from build123d import *

# Parameters (mm, degrees)
F1_DEPTH = 14.2875
F3_DEPTH = 28.576
F5_DEPTH = 38.1
F6_R     = 5.08
F7_SIZE  = 2.38125


with BuildPart() as f1:
    # F0 (on Front) → F1 (new body, symmetric)
    with BuildSketch(Plane.XZ):
        with BuildLine():
            Line((76.2, 14.2875), (41.275, 14.2875))
            Line((41.275, 14.2875), (4.333811, 1.500165))
            ThreePointArc((4.333811, 1.500165), (3.265599, 0), (4.333811, -1.500165))
            Line((4.333811, -1.500165), (41.275, -14.2875))
            Line((41.275, -14.2875), (76.2, -14.2875))
            Line((76.2, -14.2875), (114.3, -14.2875))
            Line((114.3, -14.2875), (114.3, 14.2875))
            Line((114.3, 14.2875), (76.2, 14.2875))
        make_face()
    extrude(amount=F1_DEPTH, both=True)

    # F2 (on face) → F3 (cut, through all)
    with BuildSketch(Plane.XY.offset(14.2875)):
        with BuildLine():
            Line((66.675, 6.35), (53.975, 6.35))
            ThreePointArc((53.975, 6.35), (47.625, 0), (53.975, -6.35))
            Line((53.975, -6.35), (66.675, -6.35))
            ThreePointArc((66.675, -6.35), (73.025, 0), (66.675, 6.35))
        make_face()
    extrude(amount=-F3_DEPTH, mode=Mode.SUBTRACT)

    # F4 (on face) → F5 (cut)
    with BuildSketch(Plane.YZ.offset(114.3)):
        Polygon((5.918076, 14.2875), (14.2875, 5.918076), (14.2875, 14.2875), align=None)
        Polygon((-14.2875, 5.918076), (-5.918076, 14.2875), (-14.2875, 14.2875), align=None)
        Polygon((-14.2875, -14.2875), (-5.918076, -14.2875), (-14.2875, -5.918076), align=None)
        Polygon((5.918076, -14.2875), (14.2875, -14.2875), (14.2875, -5.918076), align=None)
    extrude(amount=-F5_DEPTH, mode=Mode.SUBTRACT)

    # F6
    f6_edges = [f1.edges().sort_by_distance(p)[0] for p in [
        (76.2, -10.102788, 10.102788),
        (76.2, -10.102788, -10.102788),
        (76.2, 10.102788, -10.102788),
        (76.2, 10.102788, 10.102788),
    ]]
    fillet(f6_edges, radius=F6_R)

    # F7
    f7_edges = [f1.edges().sort_by_distance(p)[0] for p in [
        (114.3, 10.102788, -10.102788),
        (114.3, 0, -14.2875),
        (114.3, -10.102788, -10.102788),
        (114.3, -14.2875, 0),
        (114.3, -10.102788, 10.102788),
        (114.3, 0, 14.2875),
        (114.3, 10.102788, 10.102788),
        (114.3, 14.2875, 0),
    ]]
    chamfer(f7_edges, length=F7_SIZE)


solid = f1.part
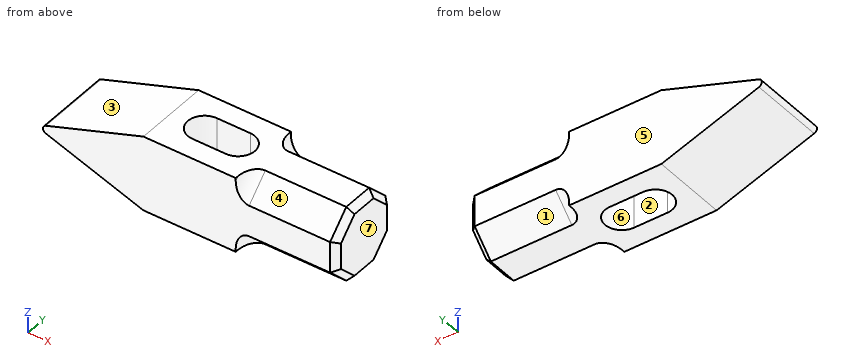
Here's how the part is built. I have some questions about the finished solid (model axes, mm). Face numbers are marked on the shaded views. A direction names the side the tool comes from. Give positions to 0.01 mm unless a question says otherwise; leave off trailing zeros. Order: outer loops, then holes, each group sorted by start corner. A loop starts at its lowest first (then second) coordinate and runs counter-clockwise, first axis right, second up. Notation, with made-up numbers: (13.5, -29) -> (32.5, -29) arc R12 ccw to (32.5, -11) -> close; hole circle Ø1 at (36.25, 33.25). An arc over 180 degrees is marked (long way). One line per item, written item: value. Start each with the question number.
1. Imagine slicing it at A-A, the plane x = 64.5. List the corners of the cut face in (y, z) for me.
2. Imagine slicing it at D-D, the plane x = 16.5. List the corners of the cut face in (y, z) for me, plus the area to 3 significant figures.
3. We'd pull the mould along X, two halves only. Please class the marked faces 5, 6 and 7: released by +X, released by -X, zero draft, split by the parting line, or undercut.
4. Will this pin go through, and if not, where does the flat tip stop? pin 1 Ø0.6 at (y, z) = (13.5, 14) entering from +X.
5. For the marked faces 1, 2, 3 and 4, which set-ups out of +Z, -Z, +X, -X, +Y, -Y let a thin tool reach every point of the face, with its end or its side?
6. I need wall thicknesses on probe 1 along Y at (x, z) = (67, -6); probe 2 along Z at (x, y) = (36, -12); probe 3 along Y at (x, z) = (51, -9.5). Which ranges of each line are inside material? Lowest first, please. Write a range as from..to.
7. Imagine slicing it at B-B, the plane y = 0. List the corners of the cut face in (x, z) for me (1 decimal), plus the area to 3 significant figures.
Values follow:
1. outline: (-14.29, -14.29) -> (-6.35, -14.29) -> (-6.35, 14.29) -> (-14.29, 14.29) -> close; (6.35, -14.29) -> (14.29, -14.29) -> (14.29, 14.29) -> (6.35, 14.29) -> close
2. outline: (-14.29, -5.71) -> (14.29, -5.71) -> (14.29, 5.71) -> (-14.29, 5.71) -> close
2. area: 326 mm2
3. face 5: zero draft
3. face 6: undercut
3. face 7: released by +X
4. pin 1: stops at x = 76.2
5. face 1: -Z, +X, +Y
5. face 2: +Z, -Z
5. face 3: +Z, -X, +Y, -Y
5. face 4: +Z, +X, -Y
6. probe 1: y = -14.29..-6.34, 6.34..14.29
6. probe 2: z = -12.46..12.46
6. probe 3: y = -14.29..-5.61, 5.61..14.29
7. outline: (4.3, -1.5) -> (41.3, -14.3) -> (47.6, -14.3) -> (47.6, 14.3) -> (41.3, 14.3) -> (4.3, 1.5) arc R1.6 ccw to start; (73, -14.3) -> (111.9, -14.3) -> (114.3, -11.9) -> (114.3, 11.9) -> (111.9, 14.3) -> (73, 14.3) -> close
7. area: 1,940 mm2
